Can you work these out from the model? Positions are in its coordinate system, mm. A direction names the side the tool comes from. Coordinates: 2 decimals unless noted, no trailing zeros. Order: outer loops, then holes, each group sorted by start corner. A loop starts at its lowest first (then second) coordinate and runs counter-clockwise, first axis right, second up. Notation, with made-up numbers: (87, 9) -> (142, 9) arc R3 ccw to (142, 14) -> close; hole circle Ø5 at (17.25, -12.75). An arc over 180 degrees is marked (long way). Answer as CSV lines item,"result".
from build123d import *

# Parameters (mm, degrees)
F0_W     = 200
F0_H     = 25
F1_DEPTH = 25
F3_DEPTH = 200.001
F5_DEPTH = 25.001


with BuildPart() as f1:
    # F0 (on Top) → F1 (new body)
    with BuildSketch(Plane.XY):
        Rectangle(F0_W, F0_H)
    extrude(amount=F1_DEPTH)

    # F2 (on face) → F3 (cut, through all)
    with BuildSketch(Plane.YZ.offset(100)):
        with BuildLine():
            ThreePointArc((0, 25), (6.470476, 24.148146), (12.5, 21.650635))
            Line((12.5, 21.650635), (12.5, 25))
            Line((12.5, 25), (0, 25))
        make_face()
        with BuildLine():
            Line((-12.5, 25), (-12.5, 21.650635))
            ThreePointArc((-12.5, 21.650635), (-6.470476, 24.148146), (0, 25))
            Line((0, 25), (-12.5, 25))
        make_face()
        with BuildLine():
            Line((12.5, 0), (12.5, 3.349365))
            ThreePointArc((12.5, 3.349365), (6.470476, 0.851854), (0, 0))
            Line((0, 0), (12.5, 0))
        make_face()
        with BuildLine():
            ThreePointArc((0, 0), (-6.470476, 0.851854), (-12.5, 3.349365))
            Line((-12.5, 3.349365), (-12.5, 0))
            Line((-12.5, 0), (0, 0))
        make_face()
    extrude(amount=-F3_DEPTH, mode=Mode.SUBTRACT)

    # F4 (on Top) → F5 (cut, through all)
    with BuildSketch(Plane.XY):
        with BuildLine():
            Line((-100, 12.5), (-100, 2.5))
            Line((-100, 2.5), (5, 2.5))
            ThreePointArc((5, 2.5), (12.071068, 5.428932), (15, 12.5))
            Line((15, 12.5), (-100, 12.5))
        make_face()
        with BuildLine():
            Line((-100, -2.5), (-100, -12.5))
            Line((-100, -12.5), (15, -12.5))
            ThreePointArc((15, -12.5), (12.071068, -5.428932), (5, -2.5))
            Line((5, -2.5), (-100, -2.5))
        make_face()
    extrude(amount=F5_DEPTH, mode=Mode.SUBTRACT)


solid = f1.part
Q1. If I drill on line 1 (Y direction, x = -43, z = 17); line 2 (Y direction, x = 48, z = 2.5); line 3 (Z direction, x = 13.5, y = -1.75), over which ranges is the centre line in solid material (lowest first)?
Solution:
line 1,"-2.5 to 2.5"
line 2,"-10.9 to 10.9"
line 3,"0.06 to 24.94"
Q2. Which directions (+Z, -Z, +X, -X, +Y, -Y) give clear straight access to the entire face, cutting with the end or side of a thin tool? Please do faces 1 (the flat face through (-48, 2.5, 12)), 2 (the flat face through (100, 0, 12)), 3 (the flat face through (-47, -2.5, 12)).
Solution:
face 1,"+Z, -Z, -X, +Y"
face 2,"+Z, -Z, +X, +Y, -Y"
face 3,"+Z, -Z, -X, -Y"
Q3. Imagine slicing it at C-C (x = 47). List the corners of the cut face in (y, z) for me.
Solution:
outline,"(-12.5, 3.35) arc R25 ccw to (0, 0) arc R25 ccw to (12.5, 3.35) -> (12.5, 21.65) arc R25 ccw to (0, 25) arc R25 ccw to (-12.5, 21.65) -> close"
Q4. Imagine slicing it at A-A (z = 7). List the corners of the cut face in (x, y) for me.
Solution:
outline,"(-100, -2.5) -> (5, -2.5) arc R10 cw to (15, -12.5) -> (100, -12.5) -> (100, 12.5) -> (15, 12.5) arc R10 cw to (5, 2.5) -> (-100, 2.5) -> close"
Q5. Imagine slicing it at D-D (y = -9.5). List the corners of the cut face in (x, z) for me.
Solution:
outline,"(14.54, 1.88) -> (100, 1.88) -> (100, 23.12) -> (14.54, 23.12) -> close"
Q6. Imagine slicing it at B-B (x = -75.5). List the corners of the cut face in (y, z) for me, and give its area (3 significant figures).
Solution:
outline,"(-2.5, 0.13) arc R25 ccw to (0, 0) arc R25 ccw to (2.5, 0.13) -> (2.5, 24.87) arc R25 ccw to (0, 25) arc R25 ccw to (-2.5, 24.87) -> close"
area,"125 mm2"
Q7. For P1, Ø7.5, axis at x = -60, z = 12, coming from the -Y side; P2, Ø3, axis at x = 72.5, y = 10, coming from the -Z side, each with a flat end and sliding along its axis, tell me the tip position at first contact or that it passes through.
Solution:
P1,"y = -2.5"
P2,"z = 1.49"
